Autodesk Inventor part; units mm, degrees
ref_plane "YZ Plane" through (0, 0, 0) normal (1, 0, 0) x (0, 1, 0)
ref_plane "XZ Plane" through (0, 0, 0) normal (0, 1, 0) x (-1, 0, 0)
ref_plane "XY Plane" through (0, 0, 0) normal (0, 0, 1) x (1, 0, 0)
sketch "Sketch1" plane through (0, 0, 0) normal (0, 0, 1) x (1, 0, 0)
  line L0 (-4.7625, -2.7496) -> (-4.7625, 2.7496)
  line L1 (-4.7625, 2.7496) -> (0, 5.4993)
  line L2 (0, 5.4993) -> (4.7625, 2.7496)
  line L3 (4.7625, 2.7496) -> (4.7625, -2.7496)
  line L4 (4.7625, -2.7496) -> (0, -5.4993)
  line L5 (0, -5.4993) -> (-4.7625, -2.7496)
  point P0 (0, 0)
  point P1 (0, 0)
  dimension "Size" = 9.525
extrude "Extrusion1" add sketch "Sketch1" along normal mid plane 82.55
sketch "Sketch3" plane through (0, 0, 41.275) normal (0, 0, 1) x (1, 0, 0)
  line L0 (-4.7625, 2.7496) -> (0, 5.4993) construction
  line L1 (0, 5.4993) -> (4.7625, 2.7496) construction
  line L2 (4.7625, 2.7496) -> (4.7625, -2.7496) construction
  line L3 (4.7625, -2.7496) -> (0, -5.4993) construction
  line L4 (0, -5.4993) -> (-4.7625, -2.7496) construction
  line L5 (-4.7625, -2.7496) -> (-4.7625, 2.7496) construction
  point P0 (0, 0)
hole "Hole1" at (0, 0, 41.275) direction (0, 0, -1) diameter 3.9624 end through all
sketch "Sketch4" plane through (0, 0, 41.275) normal (0, 0, 1) x (1, 0, 0)
  circle A0 centre (0, 0) radius 1.9812 construction
  line L0 (-4.7625, 2.7496) -> (0, 5.4993) construction
  line L1 (0, 5.4993) -> (4.7625, 2.7496) construction
  line L2 (4.7625, 2.7496) -> (4.7625, -2.7496) construction
  line L3 (4.7625, -2.7496) -> (0, -5.4993) construction
  line L4 (0, -5.4993) -> (-4.7625, -2.7496) construction
  line L5 (-4.7625, -2.7496) -> (-4.7625, 2.7496) construction
  circle A1 centre (0, 0) radius 5.1245
  circle A2 centre (0, 0) radius 8.89
  dimension "thunder" = 10.2489
  dimension "d16" = 17.78
extrude "Extrusion3" cut sketch "Sketch4" against normal through all
sketch "Sketch5" plane through (0, 0, 41.275) normal (0, 0, 1) x (1, 0, 0)
  circle A0 centre (0, 0) radius 1.9812
  circle A1 centre (0, 0) radius 4.7625
  line L0 (4.7625, -1.8917) -> (4.7625, 1.8917)
  line L1 (4.0195, 3.1786) -> (0.743, 5.0703)
  line L2 (-0.743, 5.0703) -> (-4.0195, 3.1786)
  line L3 (-4.7625, 1.8917) -> (-4.7625, -1.8917)
  line L4 (-4.0195, -3.1786) -> (-0.743, -5.0703)
  line L5 (0.743, -5.0703) -> (4.0195, -3.1786)
  circle A2 centre (0, 0) radius 1.9812
  arc A3 (4.0195, -3.1786) -> (4.7625, -1.8917) centre (0, 0) ccw
  arc A4 (4.7625, 1.8917) -> (4.0195, 3.1786) centre (0, 0) ccw
  arc A5 (0.743, 5.0703) -> (-0.743, 5.0703) centre (0, 0) ccw
  arc A6 (-4.0195, 3.1786) -> (-4.7625, 1.8917) centre (0, 0) ccw
  arc A7 (-4.7625, -1.8917) -> (-4.0195, -3.1786) centre (0, 0) ccw
  arc A8 (-0.743, -5.0703) -> (0.743, -5.0703) centre (0, 0) ccw
  point P0 (2.3813, -4.1244)
  point P1 (-2.3813, -4.1244)
  point P2 (-4.7625, 0)
  point P3 (-2.3813, 4.1244)
  point P4 (2.3812, 4.1244)
  point P5 (4.7625, 0)
  dimension "d21" = 9.525
extrude "Extrusion4" cut sketch "Sketch5" against normal blind 15.875 contours L0 A3 L5 A1 | A1 L1 A4 L0 | A1 L2 A5 L1 | L5 A8 L4 A1 | A1 L3 A6 L2 | L4 A7 L3 A1
mirror "Mirror2" about plane through (0, 0, 0) normal (0, 0, 1) of "Extrusion4"
equation "\"bearing\" = 25.4"
properties part number "GP10-012" material "Aluminum 6061"
Could you check a few things on this model? Use its own coordinates, in mm. A direction names the side the tool comes from. Coordinates: 2 decimals unless noted, no trailing zeros. Loops run counter-clockwise (first coordinate to the right, second up) from the corner with the lowest first, then second, coordinate; pieces in that order, holes last. Notation, with made-up numbers: M 75,-34.5 L 110,-34.5 A24 cw 110,2.5 Z; hole C 57,-33.5 d7. An arc over 180 degrees is marked long. Put each result on its own line as item: value. Start each with the question number.
(1) I need wall thicknesses on line 1 (X direction, y = 0, z = -21); line 2 (X direction, y = 1.25, z = 23.5); line 3 (Y direction, x = 1.5, z = 37). Which ranges of each line are inside material? Lowest first, please. Write a range as from..to.
(2) For faces 1 (the face through (4.3, -2.5, -25.4)), 2 (the face through (-4.3, 2.4, -25.4)), 3 (the face through (-3.78, 2.9, -33.45)), 4 (the face through (-4.3, -2.5, 25.4)), which set-ups out of +Z, -Z, +X, -X, +Y, -Y let a thin tool reach every point of the face, with its end or its side?
(3) Suppose I cut it at B-B on z = 32. Please give me the cut outline in (x, y) (1 decimal).
(4) Suppose I cut it at C-C on z = -2. Please give me the cut outline in (x, y).
(5) Will these pins go through, and if not, where does the flat tip stop? P1, Ø3, axis at x = -2.5, z = 15.5, coming from the +Y side; P2, Ø3, axis at x = 2, z = -22, coming from the -Y side.
Solutions:
1. line 1: x = -4.76..-1.98, 1.98..4.76
1. line 2: x = -4.76..-1.54, 1.54..4.76
1. line 3: y = -4.52..-1.29, 1.29..4.52
2. face 1: -Z, +X, -Y
2. face 2: -Z, -X, +Y
2. face 3: -Z
2. face 4: +Z, -X, -Y
3. outline: C 0,0 d9.5; hole C 0,0 d4
4. outline: M -4.76,-1.89 A5.12 ccw -4.02,-3.18 L -0.74,-5.07 A5.12 ccw 0.74,-5.07 L 4.02,-3.18 A5.12 ccw 4.76,-1.89 L 4.76,1.89 A5.12 ccw 4.02,3.18 L 0.74,5.07 A5.12 ccw -0.74,5.07 L -4.02,3.18 A5.12 ccw -4.76,1.89 Z; hole C 0,0 d3.96
5. P1: stops at y = 4.92
5. P2: stops at y = -5.1
